The model under review builds one solid part; all positions refer to its coordinate system, in mm. Face numbers are marked on the shaded views. A direction names the side the tool comes from. Give positions to 0.01 mm unless a question says otherwise; leave off trailing zeros. Loops run counter-clockwise (first coordinate to the right, second up) from the corner with the lowest first, then second, coordinate; pieces in that order, holes last. Notation, with made-up numbers: M 10,19 L 58,19 A7 cw 58,31 Z; hole C -23,8.5 d7. An arc over 180 degrees is marked long. One line per item, written item: value. Start each with the question number.
Q1. We need section D-D on z = 5. Write out the cut boundary in (x, y).
Q2. We need section B-B on z = -5.75. Write out the cut boundary in (x, y), plus the area to 3 significant figures.
Q3. We need section C-C on y = 42. Write out the cut boundary in (x, z).
Q4. For pin 1 (1 mm diameter, centred on y = 21.5, z = 1, fed in from -X); pin 2 (2 mm diameter, centred on x = -0.5, y = 33.5, fed in from +Z); pin 3 (4 mm diameter, centred on y = 38.5, z = 4, fed in from +X), all flat-tipped, find the tip position at first contact; note any pin that passes through.
Q5. We need section A-A on x = 0. Write out the cut boundary in (y, z) (3 decimals).
Q6. To check wall thickness, follow line 1 along Y through (x, z) = (-0.5, -7); line 2 along Z through (x, y) = (3.25, 40.5); line 3 along Z through (x, y) = (-0.25, 49.5). State the ranges of each line that lie inside material, in increasing order. Write a range as from..to.
Q7. For the marked faces 1, 2, 3 and 4, list the 3-axis set-ups (+Z, -Z, +X, -X, +Y, -Y) from which the entire face can be reached by the end or side of a thin tool; tool diameter is ignored.
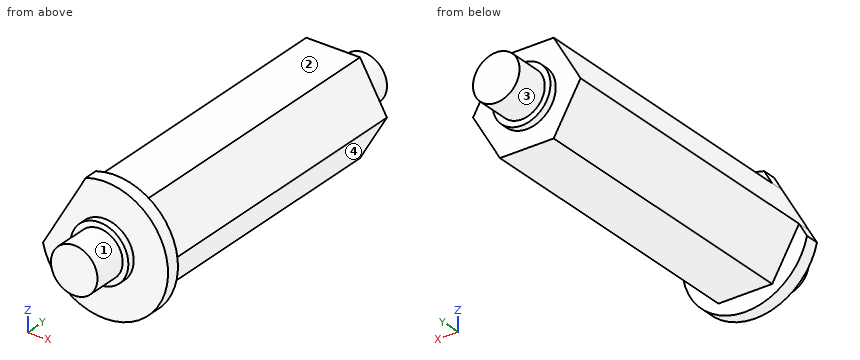
Autodesk Fusion 360 part; units mm, degrees
sketch "Sketch1" plane through (0, 0, 0) normal (0, 1, 0) x (1, 0, 0)
  circle A0 centre (0, 0) radius 3.125
  circle A1 centre (0, 0) radius 3.887
  line L0 (7.2169, 0) -> (3.6084, 6.25)
  line L1 (3.6084, 6.25) -> (-3.6084, 6.25)
  line L2 (-3.6084, 6.25) -> (-7.2169, 0)
  line L3 (-7.2169, 0) -> (-3.6084, -6.25)
  line L4 (-3.6084, -6.25) -> (3.6084, -6.25)
  line L5 (3.6084, -6.25) -> (7.2169, 0)
  line L6 (-8.2931, 1.8641) -> (-2.5322, -8.1141)
  arc A2 (-2.5322, -8.1141) -> (-8.2931, 1.8641) centre (0, 0) ccw
  dimension "d1" = 6.25
  dimension "d2" = 0.762
  dimension "d3" = 6.25
  dimension "d22" = 8.5
extrude "Extrude1" add sketch "Sketch1" along normal blind 4.572 contours A0
extrude "Extrude2" add sketch "Sketch1" along normal blind 0.9652 from surface at 4.572 contours A0 | A1
extrude "Extrude3" add sketch "Sketch1" along normal blind 41.402 from surface at 5.5372 contours A0 | A1 | L0 L1 L2 L3 L4 L5 L6
extrude "Extrude4" add sketch "Sketch1" along normal blind 0.9652 from surface at 46.9392 contours A0 | A1
extrude "Extrude5" add sketch "Sketch1" along normal blind 4.572 from surface at 47.9044 contours A0
extrude "Extrude6" add sketch "Sketch1" along normal blind 1.8 from surface at 5.5372 contours L0 L1 L2 L4 L5 L6 A2
equation "d1 = ( ( 1 / 4 ) * 1 ) * 1 in - 0.1 mm"
equation "d3 = 0.25 in - 0.1 mm"
Solved:
1. outline: M -4.33,5.54 L 6.87,5.54 L 6.87,7.34 L 4.33,7.34 L 4.33,46.94 L -4.33,46.94 Z
2. outline: M -6.26,5.54 L 6.26,5.54 L 6.26,7.34 L 3.9,7.34 L 3.9,46.94 L -3.9,46.94 L -3.9,7.34 L -6.26,7.34 Z
2. area: 331 mm2
3. outline: M -7.22,0 L -3.61,-6.25 L 3.61,-6.25 L 7.22,0 L 3.61,6.25 L -3.61,6.25 Z
4. pin 1: x = -6.93
4. pin 2: z = 6.25
4. pin 3: x = 6.06
5. outline: M 0,-3.125 L 4.572,-3.125 L 4.572,-3.887 L 5.537,-3.887 L 5.537,-8.5 L 7.337,-8.5 L 7.337,-6.25 L 46.939,-6.25 L 46.939,-3.887 L 47.904,-3.887 L 47.904,-3.125 L 52.476,-3.125 L 52.476,3.125 L 47.904,3.125 L 47.904,3.887 L 46.939,3.887 L 46.939,6.25 L 7.337,6.25 L 7.337,8.5 L 5.537,8.5 L 5.537,3.887 L 4.572,3.887 L 4.572,3.125 L 0,3.125 Z
6. line 1: 5.54..7.34
6. line 2: -6.25..6.25
6. line 3: -3.11..3.11
7. face 1: -Y
7. face 2: +Z, +X, -X, +Y
7. face 3: +Y
7. face 4: -Z, +X, +Y
